Geometry: final body of the model. Coordinates: model frame, mm. Give positions to 0.01 mm unless a question says otherwise; leave off trailing zeros. Write each loop counter-clockwise with the first axis right and the second up, starting at its lowest first coordinate (ties: lowest second). Pieces come first, ordered by that corner, then holes. Notation, with made-up numbers: M -5.75,85 L 12.25,85 A9 cw 12.25,95 Z; hole C -28.5,-13 d9. An arc over 180 degrees is marked long. Use one line per item in the form item = value. Start each with the question number.
Item 1: Section query D-D on z = 0.45. Give the number of separate pieces and of enclosed holes in the cut face, then the cut area to 3 significant figures.
Item 2: Pull-direction query (X, two-part tool) for faces 1 (the cylindrical face through (-0.521, -37.034, 0.986)), 2 (the cylindrical face through (-41.265, -31.641, 0.986)), 3 (the flat face through (11, -34, 2)); classes: released by +X, released by -X, zero draft, split by the parting line, or undercut.
Item 3: Material intervals for line 1 along Y through (x, z) = (-32, 1.6); line 2 along Y through (x, z) = (39, 0.8); line 3 along X through (y, z) = (2.5, 0.55), sorted ascending. Write a range as from..to.
Item 4: Contact query for a flat-ended pin moving along its axis: P1, Ø1, axis at y = 18, z = 1.5, coming from the -X side. Output: stop coordinate, or through.
Item 5: Section query C-C on y = 18. Return loops of the section in (x, z), then the cut area to 3 significant figures.
Item 6: Section query A-A on x = 0. Return loops of the section in (y, z), then the cut area to 3 significant figures.
Item 7: Section query B-B on y = -6. Return loops of the section in (x, z).
from build123d import *

# Parameters (mm, degrees)
F0_R     = 52
F0_R_2   = 4
F0_R_3   = 35
F1_DEPTH = 2
F2_DEPTH = 2


with BuildPart() as f1:
    # F0 (on Top) → F1 (new body)
    with BuildSketch(Plane.XY):
        Circle(F0_R)
        with Locations((-28.9913780286, -28.9913780286)):
            Circle(F0_R_2, mode=Mode.SUBTRACT)
        with Locations((-15.690020727, -37.879060833)):
            Circle(F0_R_2, mode=Mode.SUBTRACT)
        with Locations((-37.879060833, -15.690020727)):
            Circle(F0_R_2, mode=Mode.SUBTRACT)
        with Locations((0, -41)):
            Circle(F0_R_2, mode=Mode.SUBTRACT)
        with Locations((15.690020727, -37.879060833)):
            Circle(F0_R_2, mode=Mode.SUBTRACT)
        with Locations((28.9913780286, -28.9913780286)):
            Circle(F0_R_2, mode=Mode.SUBTRACT)
        with Locations((37.879060833, -15.690020727)):
            Circle(F0_R_2, mode=Mode.SUBTRACT)
        with Locations((-41, 0)):
            Circle(F0_R_2, mode=Mode.SUBTRACT)
        with Locations((-37.879060833, 15.690020727)):
            Circle(F0_R_2, mode=Mode.SUBTRACT)
        with Locations((-28.9913780286, 28.9913780286)):
            Circle(F0_R_2, mode=Mode.SUBTRACT)
        with Locations((-15.690020727, 37.879060833)):
            Circle(F0_R_2, mode=Mode.SUBTRACT)
        Circle(F0_R_3, mode=Mode.SUBTRACT)
        with Locations((41, 0)):
            Circle(F0_R_2, mode=Mode.SUBTRACT)
        with Locations((37.879060833, 15.690020727)):
            Circle(F0_R_2, mode=Mode.SUBTRACT)
        with Locations((15.690020727, 37.879060833)):
            Circle(F0_R_2, mode=Mode.SUBTRACT)
        with Locations((0, 41)):
            Circle(F0_R_2, mode=Mode.SUBTRACT)
        with Locations((28.9913780286, 28.9913780286)):
            Circle(F0_R_2, mode=Mode.SUBTRACT)
    extrude(amount=F1_DEPTH)

    # F0 (on Top) → F2 (join)
    with BuildSketch(Plane.XY):
        Circle(F0_R)
        with Locations((-28.9913780286, -28.9913780286)):
            Circle(F0_R_2, mode=Mode.SUBTRACT)
        with Locations((-15.690020727, -37.879060833)):
            Circle(F0_R_2, mode=Mode.SUBTRACT)
        with Locations((-37.879060833, -15.690020727)):
            Circle(F0_R_2, mode=Mode.SUBTRACT)
        with Locations((0, -41)):
            Circle(F0_R_2, mode=Mode.SUBTRACT)
        with Locations((15.690020727, -37.879060833)):
            Circle(F0_R_2, mode=Mode.SUBTRACT)
        with Locations((28.9913780286, -28.9913780286)):
            Circle(F0_R_2, mode=Mode.SUBTRACT)
        with Locations((37.879060833, -15.690020727)):
            Circle(F0_R_2, mode=Mode.SUBTRACT)
        with Locations((-41, 0)):
            Circle(F0_R_2, mode=Mode.SUBTRACT)
        with Locations((-37.879060833, 15.690020727)):
            Circle(F0_R_2, mode=Mode.SUBTRACT)
        with Locations((-28.9913780286, 28.9913780286)):
            Circle(F0_R_2, mode=Mode.SUBTRACT)
        with Locations((-15.690020727, 37.879060833)):
            Circle(F0_R_2, mode=Mode.SUBTRACT)
        Circle(F0_R_3, mode=Mode.SUBTRACT)
        with Locations((41, 0)):
            Circle(F0_R_2, mode=Mode.SUBTRACT)
        with Locations((37.879060833, 15.690020727)):
            Circle(F0_R_2, mode=Mode.SUBTRACT)
        with Locations((15.690020727, 37.879060833)):
            Circle(F0_R_2, mode=Mode.SUBTRACT)
        with Locations((0, 41)):
            Circle(F0_R_2, mode=Mode.SUBTRACT)
        with Locations((28.9913780286, 28.9913780286)):
            Circle(F0_R_2, mode=Mode.SUBTRACT)
    extrude(amount=F2_DEPTH)


solid = f1.part
Answer sheet:
q1.separate_pieces = 1
q1.enclosed_holes = 17
q1.area = 3,840 mm2
q2.face_1 = undercut
q2.face_2 = split by the parting line
q2.face_3 = zero draft
q3.line_1 = -40.99..-31.63, -26.36..-14.18, 14.18..26.36, 31.63..40.99
q3.line_2 = -34.39..-19.53, -11.85..-3.46, 3.46..11.85, 19.53..34.39
q3.line_3 = -51.94..-44.12, -37.88..-34.91, 34.91..37.88, 44.12..51.94
q4.P1 = -48.97
q5.outline = M -48.79,0 L -41.14,0 L -41.14,2 L -48.79,2 Z; M -34.61,0 L -30.02,0 L -30.02,2 L -34.61,2 Z; M 30.02,0 L 34.61,0 L 34.61,2 L 30.02,2 Z; M 41.14,0 L 48.79,0 L 48.79,2 L 41.14,2 Z
q5.area = 48.9 mm2
q6.outline = M -52,0 L -45,0 L -45,2 L -52,2 Z; M -37,0 L -35,0 L -35,2 L -37,2 Z; M 35,0 L 37,0 L 37,2 L 35,2 Z; M 45,0 L 52,0 L 52,2 L 45,2 Z
q6.area = 36.0 mm2
q7.outline = M -51.65,0 L -34.48,0 L -34.48,2 L -51.65,2 Z; M 34.48,0 L 51.65,0 L 51.65,2 L 34.48,2 Z
